from build123d import *

# Parameters (mm, degrees)
F0_R     = 7.9375
F1_DEPTH = 50.8
F2_R     = 8.89
F3_R     = 12.7


with BuildPart() as f1:
    # F0 (on Top) → F1 (new body)
    with BuildSketch(Plane.XY):
        Polygon((-120.983749, -69.85), (0, -139.7), (120.983749, -69.85), (324.183749, -69.85), (324.183749, -19.05), (116.475461, -19.05), (76.533749, -44.186781), (0, -88.373561), (-76.533749, -44.186781), (-76.533749, 44.186781), (0, 88.373561), (22.636533, 101.44277), (22.636533, 126.630791), (0, 139.7), (-120.983749, 69.85), align=None)
        with Locations((222.583749, -44.45)):
            Circle(F0_R, mode=Mode.SUBTRACT)
    extrude(amount=F1_DEPTH)

    # F2
    f2_edges = [f1.edges().sort_by_distance(p)[0] for p in [
        (-120.983749, 69.85, 25.4),
        (-120.983749, -69.85, 25.4),
        (0, -139.7, 25.4),
        (120.983749, -69.85, 25.4),
        (-76.533749, 44.186781, 25.4),
        (-76.533749, -44.186781, 25.4),
        (0, -88.373561, 25.4),
    ]]
    fillet(f2_edges, radius=F2_R)

    # F3
    f3_edges = [f1.edges().sort_by_distance(p)[0] for p in [
        (0, 139.7, 25.4),
        (22.636533, 101.44277, 25.4),
        (22.636533, 126.630791, 25.4),
    ]]
    fillet(f3_edges, radius=F3_R)


solid = f1.part
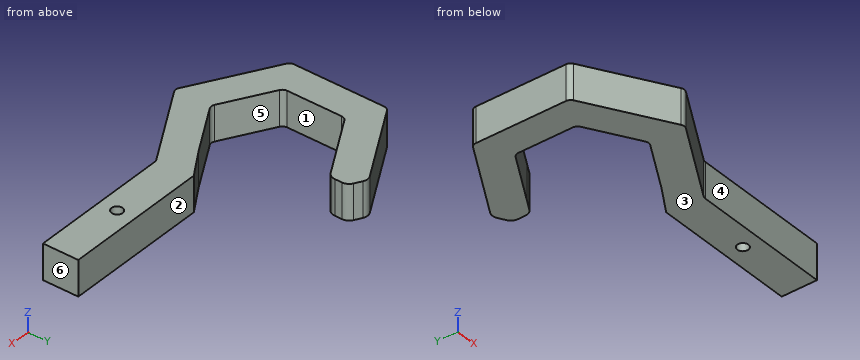
The model under review builds one solid part; all positions refer to its coordinate system, in mm. Face numbers are marked on the shaded views. A direction names the side the tool comes from. Give positions to 0.01 mm unless a question says otherwise; leave off trailing zeros. Write each loop counter-clockwise with the first axis right and the second up, starting at its lowest first coordinate (ties: lowest second). Pieces come first, ordered by that corner, then holes.
1. Add section B-B, the plane x = -55.5. Write out the cut boundary in (y, z).
2. Tool access review of the marked faces 5 and 6: name each direction out of +Z, -Z, +X, -X, +Y, -Y from which nothing blocks a thin tool from reaching the whole face with its end or side.
3. Wall thickness on L1, parallel to Y at x = 127.5, z = 15.5; L2, parallel to X at y = 1, z = 10; L3, parallel to X at y = -44, z = 39: over which ranges is each line inside the solid? List them lowest first.
4. Add section D-D, the plane x = 108. Write out the cut boundary in (y, z), plus the area to 3 significant figures.
5. Add section C-C, the plane y = -2. Write out the cut boundary in (x, z).
6. Draft analysis for pull direction Y (two halves, no side actions). For the marked faces 1, 2, 3 and 4, state which applies: +Y half, -Y half, draft (parallel to the pull), parting line (faces both ways), or undercut.
7. For P1, Ø9.5, axis at x = 222.58, y = -44.45, coming from the +Z side; P2, Ø15, axis at x = 242.5, z = 32, coming from the -Y side; P3, Ø12, axis at y = -105, z = 44.5, coming from the +X side; P4, Ø4, axis at x = 157, z = 8, coming from the +Y side, all flat-tipped, find the tip position at first contact; note any pin that passes through.
Worked answers:
1. outline: (-107.66, 0) - (-56.33, 0) - (-56.33, 50.8) - (-107.66, 50.8) - close; (56.33, 0) - (107.66, 0) - (107.66, 50.8) - (56.33, 50.8) - close
2. face 5: +Z, -Z
2. face 6: +Z, -Z, +X, +Y, -Y
3. L1: y = -69.85 to -19.05
3. L2: x = -120.98 to -76.53
3. L3: x = -120.98 to -75.03, 76.83 to 214.66, 230.51 to 324.18
4. outline: (-77.35, 0) - (-24.38, 0) - (-24.38, 50.8) - (-77.35, 50.8) - close
4. area: 2,690 mm2
5. outline: (-120.98, 0) - (-76.53, 0) - (-76.53, 50.8) - (-120.98, 50.8) - close
6. face 1: undercut
6. face 2: +Y half
6. face 3: draft
6. face 4: -Y half
7. P1: passes through
7. P2: stops at y = -69.85
7. P3: stops at x = 70.49
7. P4: stops at y = -19.05
